```python
from build123d import *

# Parameters (mm, degrees)
CYLINDER009_R          = 2.1
CYLINDER009_DEPTH      = 3
BOX018_W               = 10
BOX018_H               = 12
BOX018_DEPTH           = 3
FILLET002_R            = 4.5
FILLET003_R            = 4.5
CUT018_PLACEMENT_ANGLE = 180
CYLINDER008_R          = 2.1
CYLINDER008_DEPTH      = 3
BOX017_W               = 10
BOX017_H               = 12
BOX017_DEPTH           = 3
FILLET_R               = 4.5
FILLET001_R            = 4.5
CYLINDER002_R          = 1.3
CYLINDER002_DEPTH      = 8
BOX016_W               = 9
BOX016_H               = 10
BOX016_DEPTH           = 8
CYLINDER003_R          = 1.3
CYLINDER003_DEPTH      = 8
BOX015_W               = 12
BOX015_H               = 10
BOX015_DEPTH           = 8
CYLINDER001_R          = 1.3
CYLINDER001_DEPTH      = 8
BOX013_W               = 12
BOX013_H               = 10
BOX013_DEPTH           = 8
CYLINDER_R             = 1.3
CYLINDER_DEPTH         = 8
BOX014_W               = 12
BOX014_H               = 10
BOX014_DEPTH           = 8
BOX003_W               = 111
BOX003_H               = 69
BOX003_DEPTH           = 1
BOX002_W               = 113
BOX002_H               = 71
BOX002_DEPTH           = 1
BOX001_W               = 109
BOX001_H               = 67
BOX001_DEPTH           = 13
BOX_W                  = 113
BOX_H                  = 71
BOX_DEPTH              = 15


with BuildPart() as zylinder001:
    # Cylinder009 → Cylinder009 (new body)
    with BuildSketch(Plane(origin=(5, 5, -23), x_dir=(1, 0, 0), z_dir=(0, 0, 1))):
        Circle(CYLINDER009_R)
    extrude(amount=CYLINDER009_DEPTH)


with BuildPart() as ear_u:
    # Box018 → Box018 (new body)
    with BuildSketch(Plane(origin=(0, -3, -23), x_dir=(1, 0, 0), z_dir=(0, 0, 1))):
        with Locations((5, 6)):
            Rectangle(BOX018_W, BOX018_H)
    extrude(amount=BOX018_DEPTH)

    # Fillet002
    fillet002_edges = [ear_u.edges().sort_by_distance(p)[0] for p in [
        (10, 9, -21.5),
    ]]
    fillet(fillet002_edges, radius=FILLET002_R)

    # Fillet003
    fillet003_edges = [ear_u.edges().sort_by_distance(p)[0] for p in [
        (0, 9, -21.5),
    ]]
    fillet(fillet003_edges, radius=FILLET003_R)

    # Cut018: cut Zylinder001
    add(zylinder001.part, mode=Mode.SUBTRACT)


with BuildPart() as ear_u_1:
    # Cut018 placement: moved
    add(ear_u.part.moved(Location((62, -73, 0))).rotate(Axis((62, -73, 0), (0, 0, 1)), CUT018_PLACEMENT_ANGLE))


with BuildPart() as zylinder:
    # Cylinder008 → Cylinder008 (new body)
    with BuildSketch(Plane(origin=(5, 5, -23), x_dir=(1, 0, 0), z_dir=(0, 0, 1))):
        Circle(CYLINDER008_R)
    extrude(amount=CYLINDER008_DEPTH)


with BuildPart() as ear_o:
    # Box017 → Box017 (new body)
    with BuildSketch(Plane(origin=(0, -3, -23), x_dir=(1, 0, 0), z_dir=(0, 0, 1))):
        with Locations((5, 6)):
            Rectangle(BOX017_W, BOX017_H)
    extrude(amount=BOX017_DEPTH)

    # Fillet
    fillet_edges = [ear_o.edges().sort_by_distance(p)[0] for p in [
        (10, 9, -21.5),
    ]]
    fillet(fillet_edges, radius=FILLET_R)

    # Fillet001
    fillet001_edges = [ear_o.edges().sort_by_distance(p)[0] for p in [
        (0, 9, -21.5),
    ]]
    fillet(fillet001_edges, radius=FILLET001_R)

    # Cut017: cut Zylinder
    add(zylinder.part, mode=Mode.SUBTRACT)


with BuildPart() as ear_o_1:
    # Cut017 placement: moved
    add(ear_o.part.moved(Location((52, 0, 0))))


with BuildPart() as obj1:
    # Cylinder002 → Cylinder002 (new body)
    with BuildSketch(Plane(origin=(93.55, -8.4, -10), x_dir=(1, 0, 0), z_dir=(0, 0, 1))):
        Circle(CYLINDER002_R)
    extrude(amount=CYLINDER002_DEPTH)


with BuildPart() as obj2:
    # Box016 → Box016 (new body)
    with BuildSketch(Plane(origin=(89, -13, -10), x_dir=(1, 0, 0), z_dir=(0, 0, 1))):
        with Locations((4.5, 5)):
            Rectangle(BOX016_W, BOX016_H)
    extrude(amount=BOX016_DEPTH)

    # Cut011: cut obj1
    add(obj1.part, mode=Mode.SUBTRACT)


with BuildPart() as obj3:
    # Cylinder003 → Cylinder003 (new body)
    with BuildSketch(Plane(origin=(103.7, -64.3, -10), x_dir=(1, 0, 0), z_dir=(0, 0, 1))):
        Circle(CYLINDER003_R)
    extrude(amount=CYLINDER003_DEPTH)


with BuildPart() as obj4:
    # Box015 → Box015 (new body)
    with BuildSketch(Plane(origin=(99, -70, -10), x_dir=(1, 0, 0), z_dir=(0, 0, 1))):
        with Locations((6, 5)):
            Rectangle(BOX015_W, BOX015_H)
    extrude(amount=BOX015_DEPTH)

    # Cut012: cut obj3
    add(obj3.part, mode=Mode.SUBTRACT)


with BuildPart() as obj5:
    # Cylinder001 → Cylinder001 (new body)
    with BuildSketch(Plane(origin=(9.7, -64.3, -10), x_dir=(1, 0, 0), z_dir=(0, 0, 1))):
        Circle(CYLINDER001_R)
    extrude(amount=CYLINDER001_DEPTH)


with BuildPart() as obj6:
    # Box013 → Box013 (new body)
    with BuildSketch(Plane(origin=(2, -70, -10), x_dir=(1, 0, 0), z_dir=(0, 0, 1))):
        with Locations((6, 5)):
            Rectangle(BOX013_W, BOX013_H)
    extrude(amount=BOX013_DEPTH)

    # Cut010: cut obj5
    add(obj5.part, mode=Mode.SUBTRACT)


with BuildPart() as fasteninghole_lo:
    # Cylinder → Cylinder (new body)
    with BuildSketch(Plane(origin=(9.7, -8.4, -10), x_dir=(1, 0, 0), z_dir=(0, 0, 1))):
        Circle(CYLINDER_R)
    extrude(amount=CYLINDER_DEPTH)


with BuildPart() as fasteningblock_lo:
    # Box014 → Box014 (new body)
    with BuildSketch(Plane(origin=(2, -13, -10), x_dir=(1, 0, 0), z_dir=(0, 0, 1))):
        with Locations((6, 5)):
            Rectangle(BOX014_W, BOX014_H)
    extrude(amount=BOX014_DEPTH)

    # Cut009: cut FasteningHole_LO
    add(fasteninghole_lo.part, mode=Mode.SUBTRACT)


with BuildPart() as casebottomlip_in:
    # Box003 → Box003 (new body)
    with BuildSketch(Plane(origin=(1, -71, 3), x_dir=(1, 0, 0), z_dir=(0, 0, 1))):
        with Locations((55.5, 34.5)):
            Rectangle(BOX003_W, BOX003_H)
    extrude(amount=BOX003_DEPTH)


with BuildPart() as casebottomlip:
    # Box002 → Box002 (new body)
    with BuildSketch(Plane(origin=(0, -72, 3), x_dir=(1, 0, 0), z_dir=(0, 0, 1))):
        with Locations((56.5, 35.5)):
            Rectangle(BOX002_W, BOX002_H)
    extrude(amount=BOX002_DEPTH)

    # Cut001: cut CaseBottomLip_In
    add(casebottomlip_in.part, mode=Mode.SUBTRACT)


with BuildPart() as casebottombed_in:
    # Box001 → Box001 (new body)
    with BuildSketch(Plane(origin=(2, -70, -10), x_dir=(1, 0, 0), z_dir=(0, 0, 1))):
        with Locations((54.5, 33.5)):
            Rectangle(BOX001_W, BOX001_H)
    extrude(amount=BOX001_DEPTH)


with BuildPart() as casebottom:
    # Box → Box (new body)
    with BuildSketch(Plane(origin=(0, -72, -12), x_dir=(1, 0, 0), z_dir=(0, 0, 1))):
        with Locations((56.5, 35.5)):
            Rectangle(BOX_W, BOX_H)
    extrude(amount=BOX_DEPTH)

    # Cut: cut CaseBottomBed_In
    add(casebottombed_in.part, mode=Mode.SUBTRACT)

    # Fusion: union CaseBottomLip
    add(casebottomlip.part)

    # Fusion002: union FasteningBlock_LO
    add(fasteningblock_lo.part)

    # Fusion003: union obj6
    add(obj6.part)

    # Fusion004: union obj4
    add(obj4.part)

    # Fusion005: union obj2
    add(obj2.part)


with BuildPart() as casebottom_1:
    # Fusion005 placement: moved
    add(casebottom.part.moved(Location((0, 0, -11))))

    # Fusion010: union Ear_O
    add(ear_o_1.part)

    # Fusion011: union Ear_U
    add(ear_u_1.part)


solid = casebottom_1.part
```
Check sheet for the modelled part. Datum: model origin and axes. Units: mm. A direction names the side the tool comes from. Give positions to 0.01 mm unless a question says otherwise; leave off trailing zeros. Order: outer loops, then holes, each group sorted by start corner. A loop starts at its lowest first (then second) coordinate and runs counter-clockwise, first axis right, second up. Notation, with made-up numbers: (9.5, -33) -> (45.5, -33) arc R30 ccw to (45.5, 1) -> close; hole circle Ø2 at (34.25, -18.75). An arc over 180 degrees is marked (long way). Use CSV: the item, a comma, the result in double quotes. Start each with the question number.
1) Sectioned sample at D-D, the plane z = -9.75. Record the boundary of the cut face in (x, y).
2) Sectioned sample at A-A, the plane z = -17.75. Record the boundary of the cut face in (x, y), plus the area to 3 significant figures.
3) Go/stop test with flat-tipped pins: P1, Ø3, axis at x = 32, z = -9, coming from the +Y side; P2, Ø2.5, axis at x = 93.55, y = -8.4, coming from the +Z side; P3, Ø7, axis at x = 93, y = -8, coming from the +Z side. Record where each tip stops, or that it passes through.
4) Sectioned sample at C-C, the plane x = 17. Record the boundary of the cut face in (y, z), plus the area to 3 significant figures.
5) Material ranges on line 1 (Y direction, x = 9.7, z = -18); line 2 (X direction, y = -64.3, z = -18.75); line 3 (X direction, y = -56, z = -18), recorded low to high. Write a range as from..to.
6) Sectioned sample at B-B, the plane y = -39. Record the boundary of the cut face in (x, z).
7) Mould release check, pull along Y, two halves, no side actions. Record for faces 4 (the face through (56, -36, -21)), 5 (the face through (57, -37, -23)), 6 (the face through (60.647, -80.717, -21.479)): released by +Y, released by -Y, zero draft, split by the parting line, or undercut.
8) Set-up check for faces 1 (the face through (62, 2, -22)), 2 (the face through (55.06, -77.2, -21.52)), 3 (the face through (2, -37, -15)): record each of +Z, -Z, +X, -X, +Y, -Y from which the full face is reachable in a straight line by a thin tool's end or side.
Recorded:
1,outline,"(0, -72) -> (113, -72) -> (113, -1) -> (0, -1) -> close; hole (2, -70) -> (111, -70) -> (111, -3) -> (2, -3) -> close"
2,outline,"(0, -72) -> (113, -72) -> (113, -1) -> (0, -1) -> close; hole (2, -60) -> (14, -60) -> (14, -70) -> (99, -70) -> (99, -60) -> (111, -60) -> (111, -3) -> (98, -3) -> (98, -13) -> (89, -13) -> (89, -3) -> (14, -3) -> (14, -13) -> (2, -13) -> close; hole circle Ø2.6 at (9.7, -64.3); hole circle Ø2.6 at (9.7, -8.4); hole circle Ø2.6 at (93.55, -8.4); hole circle Ø2.6 at (103.7, -64.3)"
2,area,"1,150 mm2"
3,P1,"y = -1"
3,P2,"z = -21"
3,P3,"z = -13"
4,outline,"(-72, -23) -> (-1, -23) -> (-1, -7) -> (-2, -7) -> (-2, -8) -> (-3, -8) -> (-3, -21) -> (-70, -21) -> (-70, -8) -> (-71, -8) -> (-71, -7) -> (-72, -7) -> close"
4,area,"196 mm2"
5,line 1,"-72..-65.6, -63..-60, -13..-9.7, -7.1..-1"
5,line 2,"0..8.4, 11..14, 99..102.4, 105..113"
5,line 3,"0..2, 111..113"
6,outline,"(0, -23) -> (113, -23) -> (113, -7) -> (112, -7) -> (112, -8) -> (111, -8) -> (111, -21) -> (2, -21) -> (2, -8) -> (1, -8) -> (1, -7) -> (0, -7) -> close"
7,face 4,"undercut"
7,face 5,"zero draft"
7,face 6,"released by -Y"
8,face 1,"+Z, -Z, +X, +Y"
8,face 2,"+Z, -Z"
8,face 3,"+Z"
